Design review of the part built by this model. Coordinates are the model's own, in mm. Face numbers are marked on the shaded views. A direction names the side the tool comes from. Coordinates: 2 decimals unless noted, no trailing zeros. Loops run counter-clockwise (first coordinate to the right, second up) from the corner with the lowest first, then second, coordinate; pieces in that order, holes last. Notation, with made-up numbers: M 63.25,-33.5 L 95.25,-33.5 A15 ccw 95.25,-24.5 Z; hole C 47,-9 d4. An arc over 180 degrees is marked long. Answer as CSV lines item,"result". Start each with the question number.
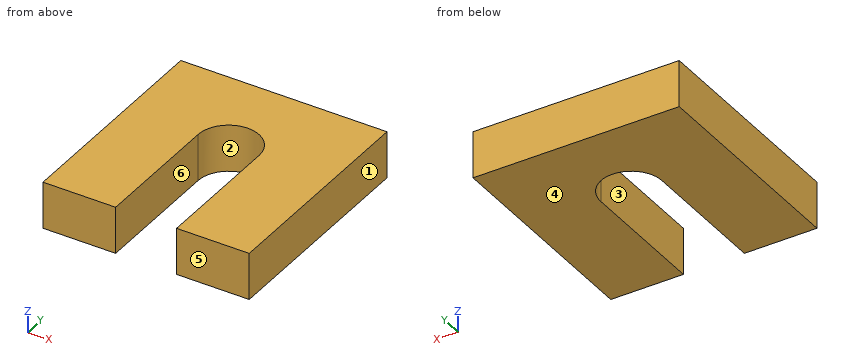
from build123d import *

# Parameters (mm, degrees)
SKETCH2_W           = 44
SKETCH2_H           = 47
BOSS_EXTRUDE1_DEPTH = 10
CUT_EXTRUDE1_DEPTH  = 10


with BuildPart() as part:
    # Sketch2 → Boss-Extrude1 (new body)
    with BuildSketch(Plane.XY):
        Rectangle(SKETCH2_W, SKETCH2_H)
    extrude(amount=BOSS_EXTRUDE1_DEPTH)

    # Sketch3 → Cut-Extrude1 (cut)
    with BuildSketch(Plane.XY.offset(10)):
        with BuildLine():
            Line((-6.5, -23.5), (-6.5, 4.628280517))
            ThreePointArc((-6.5, 4.628280517), (0, 11.128280517), (6.5, 4.628280517))
            Line((6.5, 4.628280517), (6.5, -23.5))
            ThreePointArc((6.5, -23.5), (0, -30), (-6.5, -23.5))
        make_face()
    extrude(amount=-CUT_EXTRUDE1_DEPTH, mode=Mode.SUBTRACT)


solid = part.part
Item 1: Add section B-B (z = 3). Give the boundary of the cut face in (x, y).
Item 2: Add section C-C (x = 1.5). Give the boundary of the cut face in (y, z), plus the area to 3 significant figures.
Item 3: For pin 1 (1 mm diameter, centred on x = -5.5, z = 3.5, fed in from -Y), flat-tipped, find the tip position at first contact; note if it passes through.
Item 4: Add section A-A (y = -9.5). Give the boundary of the cut face in (x, z).
Item 5: For the marked faces 5 and 6, list the 3-axis set-ups (+Z, -Z, +X, -X, +Y, -Y) from which the entire face can be reached by the end or side of a thin tool; tool diameter is ignored.
Item 6: Mouldability with a two-part tool opening along X and no side actions: class the marked faces 1, 2, 3 and 4 as released by +X, released by -X, zero draft, split by the parting line, or undercut.
Item 7: For line 1 along X through (y, z) = (-11, 4); line 2 along X through (y, z) = (9.5, 2.5); line 3 along Y through (x, z) = (4.5, 5.75), list the stretches that pass through material, from the lowest coordinate up. Write a range as from..to.
Response:
1,outline,"M -22,-23.5 L -6.5,-23.5 L -6.5,4.63 A6.5 cw 6.5,4.63 L 6.5,-23.5 L 22,-23.5 L 22,23.5 L -22,23.5 Z"
2,outline,"M 10.95,0 L 23.5,0 L 23.5,10 L 10.95,10 Z"
2,area,"125 mm²"
3,pin 1,"y = 7.13"
4,outline,"M -22,0 L -6.5,0 L -6.5,10 L -22,10 Z; M 6.5,0 L 22,0 L 22,10 L 6.5,10 Z"
5,face 5,"+Z, -Z, +X, -X, -Y"
5,face 6,"+Z, -Z, -Y"
6,face 1,"released by +X"
6,face 2,"undercut"
6,face 3,"undercut"
6,face 4,"zero draft"
7,line 1,"-22..-6.5, 6.5..22"
7,line 2,"-22..-4.3, 4.3..22"
7,line 3,"9.32..23.5"
